The figure shows three views and two pictorial views of one solid part (mm, origin at its lowest corner). Answer the questions. Coordinates: 2 decimals unless noted, no trailing zeros. Order: outer loops, then holes, each group sorted by start corner. A loop starts at its lowest first (then second) coordinate and runs counter-clockwise, first axis right, second up. Notation, with made-up numbers: (79.25, 34) -> (91.25, 34) arc R24 cw to (91.25, 56) -> close; hole circle Ø5 at (74.25, 3.25). An arc over 180 degrees is marked (long way). Use one line per item in the form item = value.
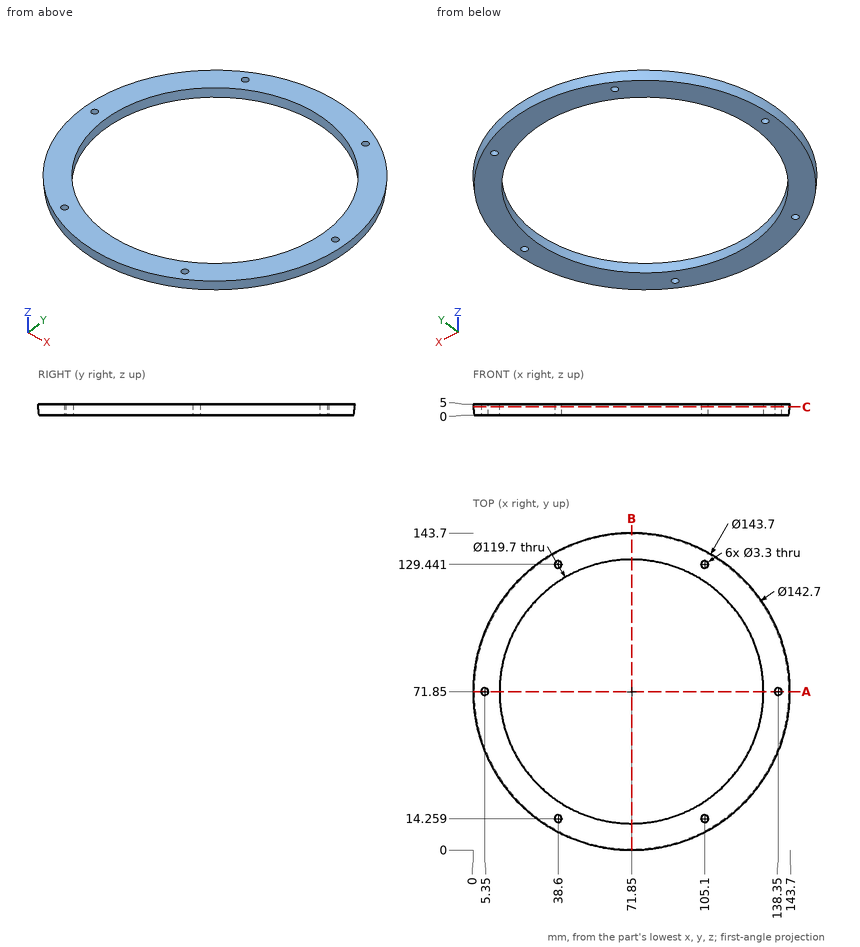
(1) Each of these flat-tipped pins is pushed along its axis until it touches: P1, Ø2, axis at y = 112.5, z = 1, coming from the +X side; P2, Ø1, axis at y = 34, z = 1.5, coming from the +X side (1 decimal); P3, Ø1, axis at x = 64, z = 2.5, coming from the +Y side. Where does it stop, or does it pass through?
Data:
P1 = 131.3
P2 = 132.8
P3 = 143.09
(2) Section B-B on x = 71.85 is taken. Write down the section's boundary in (y, z).
Data:
outline = (0, 5) -> (0.5, 0) -> (12, 0) -> (12, 5) -> close; (131.7, 0) -> (143.2, 0) -> (143.7, 5) -> (131.7, 5) -> close
(3) Section C-C on z = 3.65 is taken. Count the separate pieces of the cut face and the enclosed holes in it, plus the area to 3 significant figures.
Data:
separate_pieces = 1
enclosed_holes = 7
area = 4,850 mm²
(4) Section A-A on y = 71.85 is taken. Write down the section's boundary in (x, z), plus the area to 3 significant figures.
Data:
outline = (0, 5) -> (0.5, 0) -> (3.7, 0) -> (3.7, 5) -> close; (7, 0) -> (12, 0) -> (12, 5) -> (7, 5) -> close; (131.7, 0) -> (136.7, 0) -> (136.7, 5) -> (131.7, 5) -> close; (140, 0) -> (143.2, 0) -> (143.7, 5) -> (140, 5) -> close
area = 84.5 mm²
(5) Straight lines are drawn through the part: line 1 along X through (y, z) = (95, 3.85); line 2 along Y through (x, z) = (38, 2.4) (1 decimal); line 3 along X through (y, z) = (27, 2.15). For each, find the intervals that lie inside material, in ascending order.
Data:
line_1 = 3.95 to 16.66, 127.04 to 139.75
line_2 = 8.8 to 12.7, 15.8 to 22.5, 121.2 to 127.9, 131 to 134.9
line_3 = 16.08 to 32.22, 111.48 to 127.62
